Part print with two shaded views. Sizes in mm from the minimum x, y, z corner. Give positions to 0.01 mm unless a question says otherwise; leave off trailing zeros. Order: outer loops, then holes, each group sorted by start corner. A loop starts at its lowest first (then second) coordinate and runs counter-clockwise, first axis right, second up. Notation, with made-up numbers: (4, 32) -> (58, 32) arc R20 cw to (58, 40) -> close; hole circle Ø10 at (-33.75, -4). An arc over 180 degrees is marked (long way). Answer as CSV lines item,"result".
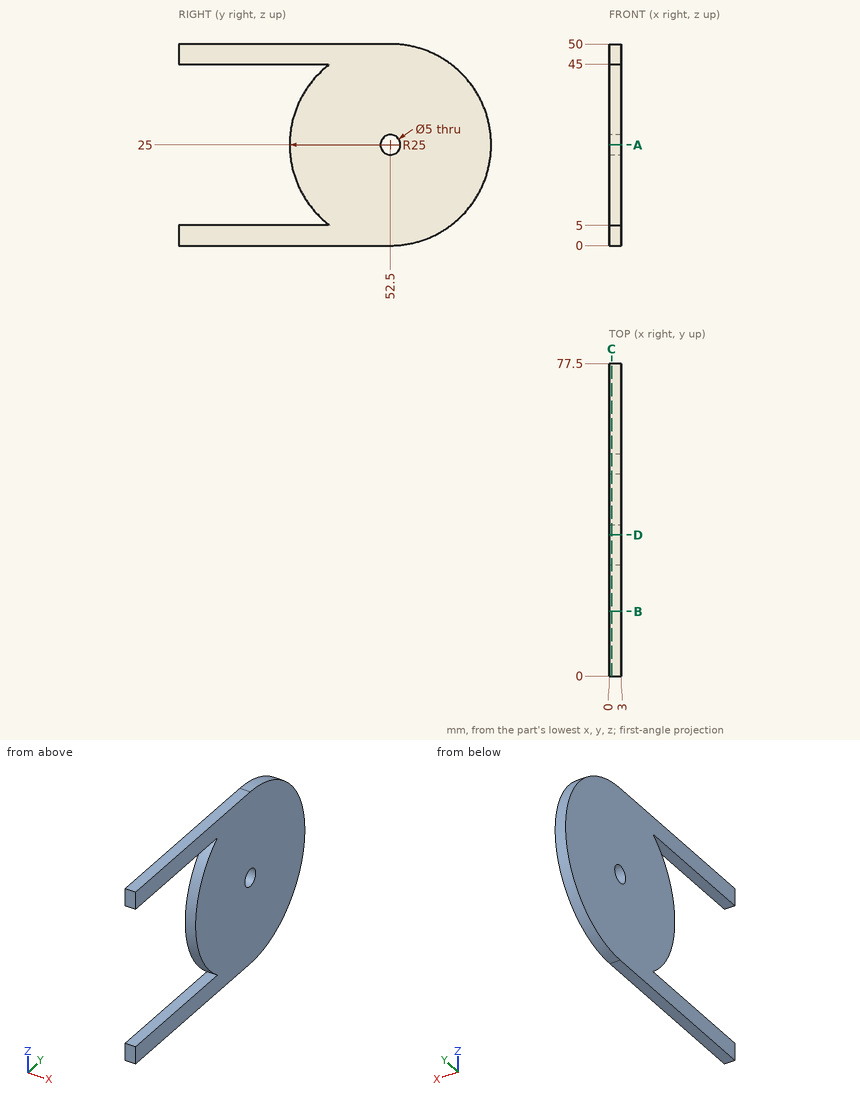
1) Band-saw the part on A-A, the plane z = 25. Write the cut outline in (x, y).
Data:
outline,"(0, 27.5) -> (3, 27.5) -> (3, 50) -> (0, 50) -> close; (0, 55) -> (3, 55) -> (3, 77.5) -> (0, 77.5) -> close"
2) Pin check, flat tips, straight feed: P1, Ø1, axis at x = 0.5, z = 40.5, coming from the -Y side; P2, Ø1.5, axis at x = 2.5, z = 33.5, coming from the +Y side. Stop position of each tip, or through.
Data:
P1,"stops at y = 32.5"
P2,"stops at y = 76.27"
3) Band-saw the part on C-C, the plane x = 0.6. Write the cut outline in (y, z), then the cut area to 3 significant figures.
Data:
outline,"(0, 0) -> (52.5, 0) arc R25 ccw to (52.5, 50) -> (0, 50) -> (0, 45) -> (37.5, 45) arc R25 ccw to (37.5, 5) -> (0, 5) -> close; hole circle Ø5 at (52.5, 25)"
area,"2,370 mm2"
4) Wall check: line 1 along Z through (x, y) = (1.8, 15.5); line 2 along Z through (x, y) = (0.9, 29.5); line 3 along Y through (x, z) = (2.25, 25). Give the ranges that are in metal, low to high. Write a range as [from, to].
Data:
line 1,"z = [0, 5], [45, 50]"
line 2,"z = [0, 5], [15.2, 34.8], [45, 50]"
line 3,"y = [27.5, 50], [55, 77.5]"
5) Band-saw the part on B-B, the plane y = 16. Write the cut outline in (x, z).
Data:
outline,"(0, 0) -> (3, 0) -> (3, 5) -> (0, 5) -> close; (0, 45) -> (3, 45) -> (3, 50) -> (0, 50) -> close"
6) Band-saw the part on D-D, the plane y = 35. Write the cut outline in (x, z).
Data:
outline,"(0, 0) -> (3, 0) -> (3, 5) -> (0, 5) -> close; (0, 7.15) -> (3, 7.15) -> (3, 42.85) -> (0, 42.85) -> close; (0, 45) -> (3, 45) -> (3, 50) -> (0, 50) -> close"
